Here's how the part is built. I have some questions about the finished solid (model axes, mm). A direction names the side the tool comes from. Round coordinates to 2 decimals unless told otherwise and drop trailing zeros. Loops run counter-clockwise (first coordinate to the right, second up) from the corner with the lowest first, then second, coordinate; pieces in that order, holes last. Notation, with made-up numbers: (87.5, 54.25) - (98.5, 54.25) arc R26 cw to (98.5, 83.25) - close; hole circle Ø10 at (56, 24). An arc over 180 degrees is marked (long way). Answer as a JSON object with one key per item and string values. Group by question number.
1) I want a section at A-A, the plane y = 10.5. Please give me the cut outline in (x, z), then the cut area to 4 significant figures.
2) If I drill on line 1 along Y through (x, z) = (21.1, 4) (3 decimals); line 2 along Y through (x, z) = (16, 1.5); line 3 along X through (y, z) = (25, 4.25), over which ranges is the centre line in solid material (lowest first)? Write a range as [from, to].
3) If we mould it in two halves opening along Y, with no side actions, what happens to faces 1 (the face through (21, 22, 0)), 2 (the face through (21, 54.1, 4)), 3 (the face through (21, 2.1, 4)), 4 (the face through (22.65, 14.93, 5.06))? For each: pulls with the +Y half, pulls with the -Y half, needs draft (parallel to the pull), parting line crosses it, or undercut.
4) I want a section at C-C, the plane z = 9. Please give me the cut outline in (x, y) (3 decimals).
5) Will these pins go through, and if not, where does the flat tip stop? P1, Ø1.7, axis at x = 21.5, y = 16.5, coming from the +Z side; P2, Ø2, axis at x = 15, z = 5, coming from the +Y side; P3, Ø3.5, axis at x = 22, y = 49, coming from the +Z side.
6) I want a section at B-B, the plane x = 9.5. Please give me the cut outline in (y, z).
7) Which directions (+Z, -Z, +X, -X, +Y, -Y) give clear straight access to the entire face, cutting with the end or side of a thin tool? Please do faces 5 (the face through (2.1, 28, 4)), 6 (the face through (40.1, 28, 4)), 7 (the face through (38.1, 28, 4)), 8 (the face through (7.6, 37, 1)).
Autodesk Inventor part; units mm, degrees
ref_plane "YZ Plane" through (0, 0, 0) normal (1, 0, 0) x (0, 1, 0)
ref_plane "XZ Plane" through (0, 0, 0) normal (0, 1, 0) x (-1, 0, 0)
ref_plane "XY Plane" through (0, 0, 0) normal (0, 0, 1) x (1, 0, 0)
sketch "Sketch2" plane through (0, 0, 0) normal (0, 0, 1) x (1, 0, 0)
  line L0 (0, 0) -> (42.2, 0)
  line L1 (42.2, 0) -> (42.2, 56.2)
  line L2 (42.2, 56.2) -> (0, 56.2)
  line L3 (0, 56.2) -> (0, 0)
  dimension "d0" = 42.2
  dimension "d1" = 56.2
extrude "Extrusion1" add sketch "Sketch2" along normal blind 2
sketch "Sketch4" plane through (0, 0, 2) normal (0, 0, 1) x (1, 0, 0)
  line L0 (2.1, 2.1) -> (40.1, 2.1)
  line L1 (40.1, 2.1) -> (40.1, 54.1)
  line L2 (40.1, 54.1) -> (2.1, 54.1)
  line L3 (2.1, 54.1) -> (2.1, 2.1)
  line L4 (42.2, 0) -> (42.2, 56.2)
  line L5 (0, 56.2) -> (0, 0)
  line L6 (0, 0) -> (42.2, 0)
  line L7 (42.2, 56.2) -> (0, 56.2)
  dimension "d12" = 38
  dimension "d13" = 52
  dimension "d49" = 42.2
  dimension "d50" = 56.2
  dimension "d51" = 2.1
  dimension "d52" = 2.1
extrude "Extrusion2" add sketch "Sketch4" along normal blind 4 contours L3 L2 L1 L0
sketch "Sketch5" plane through (0, 0, 6) normal (0, 0, 1) x (1, 0, 0)
  line L0 (4.1, 4.1) -> (38.1, 4.1)
  line L1 (38.1, 4.1) -> (38.1, 52.1)
  line L2 (38.1, 52.1) -> (4.1, 52.1)
  line L3 (4.1, 52.1) -> (4.1, 4.1)
  line L4 (40.1, 2.1) -> (40.1, 54.1)
  line L5 (2.1, 54.1) -> (2.1, 2.1)
  line L6 (2.1, 2.1) -> (40.1, 2.1)
  line L7 (40.1, 54.1) -> (2.1, 54.1)
  point P0 (0, 0)
  dimension "d16" = 34
  dimension "d17" = 48
  dimension "d45" = 38
  dimension "d46" = 2
  dimension "d47" = 52
  dimension "d48" = 2
extrude "Extrusion3" cut sketch "Sketch5" against normal blind 4 contours L3 L2 L1 L0
sketch "Sketch6" plane through (0, 0, 2) normal (0, 0, 1) x (1, 0, 0)
  line L0 (7.6, 27.1) -> (34.6, 27.1)
  line L1 (34.6, 27.1) -> (34.6, 46.6)
  line L2 (34.6, 46.6) -> (7.6, 46.6)
  line L3 (7.6, 46.6) -> (7.6, 27.1)
  line L4 (15.1, 50.6) -> (27.1, 50.6)
  line L5 (27.1, 50.6) -> (27.1, 47.6)
  line L6 (27.1, 47.6) -> (15.1, 47.6)
  line L7 (15.1, 47.6) -> (15.1, 50.6)
  line L8 (4.1, 52.1) -> (38.1, 52.1)
  line L9 (38.1, 52.1) -> (38.1, 4.1)
  line L10 (4.1, 4.1) -> (4.1, 52.1)
  point P0 (0, 0)
  dimension "d20" = 27
  dimension "d21" = 19.5
  dimension "d22" = 12
  dimension "d23" = 3
  dimension "d24" = 1
  dimension "d25" = 1.5
  dimension "d42" = 34
  dimension "d43" = 3.5
  dimension "d44" = 11
extrude "Extrusion4" cut sketch "Sketch6" against normal blind 1 contours L4 L5 L6 L7
extrude "Extrusion5" cut sketch "Sketch6" against normal blind 2 contours L3 L2 L1 L0
sketch "Sketch7" plane through (0, 0, 2) normal (0, 0, 1) x (1, 0, 0)
  circle A0 centre (21.1, 17.35) radius 2.875
  circle A1 centre (21.1, 17.35) radius 4.25
  line L0 (38.1, 4.1) -> (4.1, 4.1)
  line L1 (34.6, 27.1) -> (7.6, 27.1)
  line L2 (38.1, 52.1) -> (38.1, 4.1)
  line L3 (4.1, 4.1) -> (4.1, 52.1)
  point P0 (0, 0)
  dimension "d30" = 5.75
  dimension "d31" = 8.5
  dimension "d32" = 9
  dimension "d37" = 5.5
  dimension "d39" = 34
  dimension "d40" = 17
extrude "Extrusion6" add sketch "Sketch7" along normal blind 8
extrude "Extrusion7" cut sketch "Sketch7" against normal blind 1.75 contours A0
fillet "Fillet2" radius 1 3 edges at (21.1, 56.2, 0) (42.2, 28.1, 0) (0, 28.1, 0)
fillet "Fillet3" radius 2 4 edges at (0, 56.2, 1.5) (0.2929, 55.9071, 0.2929) (42.2, 56.2, 1.5) (41.9071, 55.9071, 0.2929)
equation "\"d51\" = -0.5 * d12 + 0.5 * d49"
equation "\"d52\" = -0.5 * d13 + 0.5 * d50"
equation "\"d46\" = -0.5 * d16 + 0.5 * d45"
equation "\"d48\" = -0.5 * d17 + 0.5 * d47"
equation "\"d43\" = -0.5 * d20 + 0.5 * d42"
equation "\"d44\" = -0.5 * d22 + 0.5 * d42"
equation "\"d40\" = 0.5 * d39"
properties part number "Enclosure v2" material "PLA Plastic"
Outcome:
{
 "1": {"outline": "(0, 1) arc R1 ccw to (1, 0) - (41.2, 0) arc R1 ccw to (42.2, 1) - (42.2, 2) - (40.1, 2) - (40.1, 6) - (38.1, 6) - (38.1, 2) - (4.1, 2) - (4.1, 6) - (2.1, 6) - (2.1, 2) - (0, 2) - close", "area": "100.0 mm^2"},
 "2": {"line 1": "[2.1, 4.1], [13.1, 14.475], [20.225, 21.6], [52.1, 54.1]", "line 2": "[0, 27.1], [46.6, 47.6], [50.6, 56.2]", "line 3": "[2.1, 4.1], [38.1, 40.1]"},
 "3": {"face 1": "needs draft", "face 2": "pulls with the +Y half", "face 3": "pulls with the -Y half", "face 4": "undercut"},
 "4": {"outline": "circle Ø8.5 at (21.1, 17.35); hole circle Ø5.75 at (21.1, 17.35)"},
 "5": {"P1": "z = 0.25", "P2": "y = 54.1", "P3": "z = 2"},
 "6": {"outline": "(0, 0) - (27.1, 0) - (27.1, 2) - (4.1, 2) - (4.1, 6) - (2.1, 6) - (2.1, 2) - (0, 2) - close; (46.6, 0) - (55.2, 0) arc R1 ccw to (56.2, 1) - (56.2, 2) - (54.1, 2) - (54.1, 6) - (52.1, 6) - (52.1, 2) - (46.6, 2) - close"},
 "7": {"face 5": "+Z, -X, +Y, -Y", "face 6": "+Z, +X, +Y, -Y", "face 7": "+Z", "face 8": "+Z, -Z"}
}
